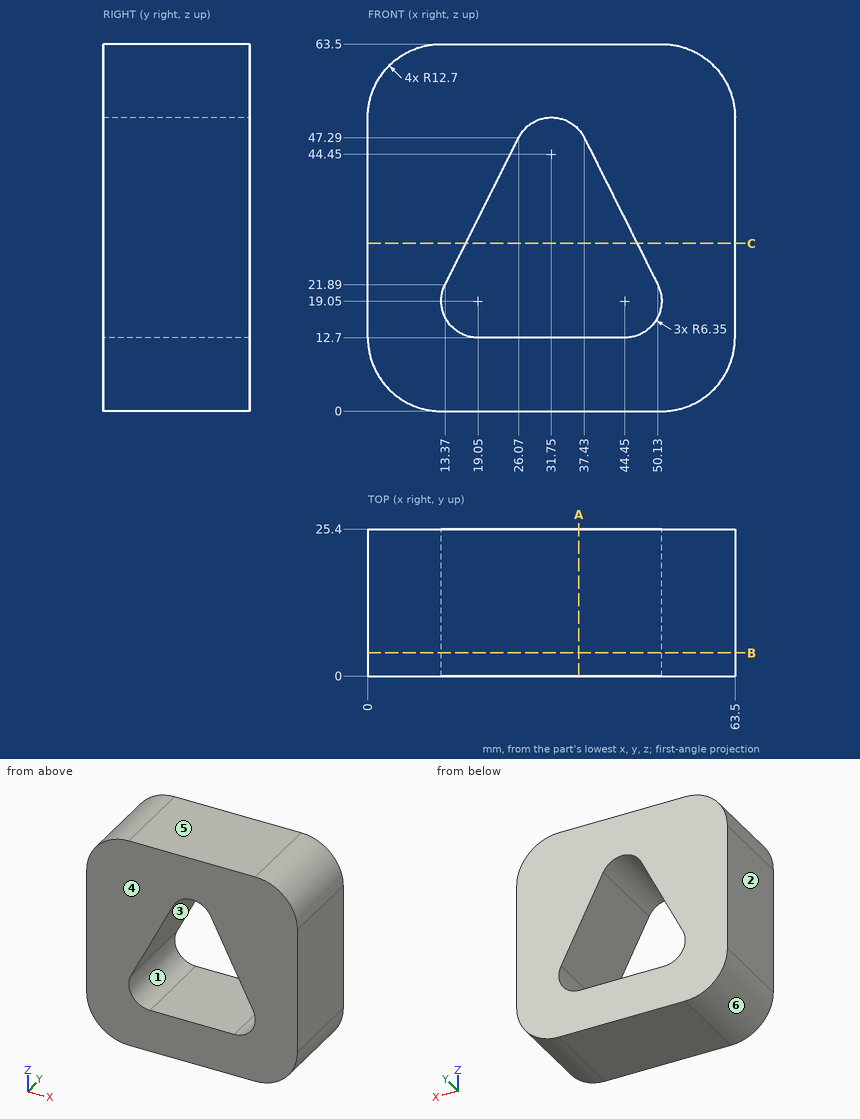
Can you work these out from the drawing? Everything is in mm from the part's minimum corner. A direction names the side the tool comes from. Round coordinates to 2 decimals unless told otherwise and drop trailing zeros. Loops run counter-clockwise (first coordinate to the right, second up) from the corner with the lowest first, then second, coordinate; pieces in that order, holes last. Notation, with made-up numbers: (-20.5, 66.5) -> (4.5, 66.5) arc R19 ccw to (4.5, 73.5) -> close; hole circle Ø10 at (-15, 55.25). An arc over 180 degrees is marked (long way). Use CSV: the item, a comma, the result in double quotes.
(1) If we mould it in two halves opening along Z, with no side actions, what happens to the marked faces 3, 4, 5 and 6? For each: +Z half, -Z half, draft (parallel to the pull), parting line (faces both ways), or undercut.
Return value:
face 3,"undercut"
face 4,"draft"
face 5,"+Z half"
face 6,"-Z half"
(2) For the marked faces 1 and 2, which set-ups out of +Z, -Z, +X, -X, +Y, -Y let a thin tool reach every point of the face, with its end or its side?
Return value:
face 1,"+Y, -Y"
face 2,"+Z, -Z, -X, +Y, -Y"
(3) If I drill on probe 1 along Z at (x, y) = (23.5, 6); probe 2 along Z at (x, y) = (20, 10.5); probe 3 along X at (y, z) = (12.5, 21), over which ranges is the centre line in solid material (lowest first)? Write a range as [from, to].
Return value:
probe 1,"z = [0, 12.7], [42.15, 63.5]"
probe 2,"z = [0, 12.7], [35.15, 63.5]"
probe 3,"x = [0, 13.01], [50.49, 63.5]"
(4) Suppose I cut it at A-A on x = 36.5. Write out the boundary of the cut face in (y, z) (1 decimal).
Return value:
outline,"(0, 0) -> (25.4, 0) -> (25.4, 12.7) -> (0, 12.7) -> close; (0, 48.7) -> (25.4, 48.7) -> (25.4, 63.5) -> (0, 63.5) -> close"
(5) Suppose I cut it at B-B on y = 4. Write out the boundary of the cut face in (x, z), plus the area to 3 significant figures.
Return value:
outline,"(0, 12.7) arc R12.7 ccw to (12.7, 0) -> (50.8, 0) arc R12.7 ccw to (63.5, 12.7) -> (63.5, 50.8) arc R12.7 ccw to (50.8, 63.5) -> (12.7, 63.5) arc R12.7 ccw to (0, 50.8) -> close; hole (13.37, 21.89) arc R6.35 ccw to (19.05, 12.7) -> (44.45, 12.7) arc R6.35 ccw to (50.13, 21.89) -> (37.43, 47.29) arc R6.35 ccw to (26.07, 47.29) -> close"
area,"2,920 mm²"
(6) Suppose I cut it at C-C on z = 29. Write out the boundary of the cut face in (x, y) (1 decimal), plus the area to 3 significant figures.
Return value:
outline,"(0, 0) -> (16.9, 0) -> (16.9, 25.4) -> (0, 25.4) -> close; (46.6, 0) -> (63.5, 0) -> (63.5, 25.4) -> (46.6, 25.4) -> close"
area,"860 mm²"
